Read the model definition and answer for the solid it produces. Units are mm, in the model's axes. Coordinates: 2 decimals unless noted, no trailing zeros. Order: outer loops, then holes, each group sorted by start corner. A loop starts at its lowest first (then second) coordinate and runs counter-clockwise, first axis right, second up.
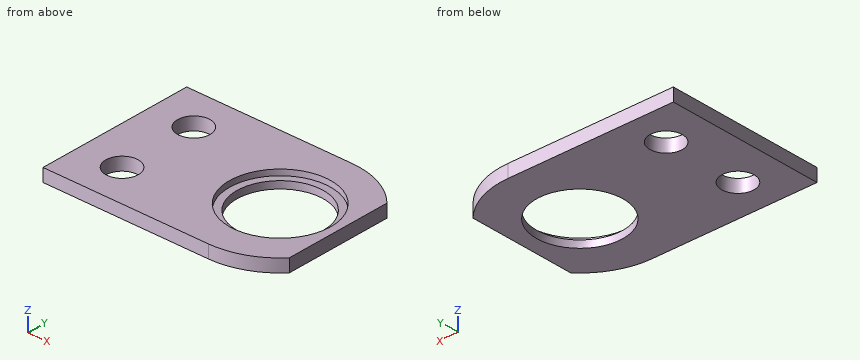
```python
from build123d import *

# Parameters (mm, degrees)
SKETCH_1_R          = 2.25
SKETCH_1_R_2        = 6
EXTRUDE_1_DEPTH     = 1.8
SKETCH_2_R          = 7
CUT_EXTRUDE_1_DEPTH = 0.8


with BuildPart() as part:
    # 草图1 → 凸台-拉伸1 (new body)
    with BuildSketch(Plane.XY):
        with BuildLine():
            Line((0, 7.478796414), (0, -7.478796414))
            ThreePointArc((0, -7.478796414), (-3.665697116, -10.081338219), (-8.066449293, -11))
            Line((-8.066449293, -11), (-31.066449293, -11))
            Line((-31.066449293, -11), (-31.066449293, 11))
            Line((-31.066449293, 11), (-8.066449293, 11))
            ThreePointArc((-8.066449293, 11), (-3.665697116, 10.081338219), (0, 7.478796414))
        make_face()
        with Locations((-25.066449293, 5.5)):
            Circle(SKETCH_1_R, mode=Mode.SUBTRACT)
        with Locations((-25.066449293, -5.5)):
            Circle(SKETCH_1_R, mode=Mode.SUBTRACT)
        with Locations((-8.066449293, 0)):
            Circle(SKETCH_1_R_2, mode=Mode.SUBTRACT)
    extrude(amount=EXTRUDE_1_DEPTH)

    # 草图2 → 切除-拉伸1 (cut)
    with BuildSketch(Plane.XY.offset(1.8)):
        with Locations((-8.066449293, 0)):
            Circle(SKETCH_2_R)
    extrude(amount=-CUT_EXTRUDE_1_DEPTH, mode=Mode.SUBTRACT)


solid = part.part
```
1) A cutting plane is placed at D-D, the plane y = 5. Determine the outline of the cut face in (x, z).
A:
outline: (-31.07, 0) - (-27.26, 0) - (-27.26, 1.8) - (-31.07, 1.8) - close; (-22.87, 0) - (-11.38, 0) - (-11.38, 1) - (-12.97, 1) - (-12.97, 1.8) - (-22.87, 1.8) - close; (-4.75, 0) - (0, 0) - (0, 1.8) - (-3.17, 1.8) - (-3.17, 1) - (-4.75, 1) - close
2) Straight lines are drawn through the part: line 1 (Y direction, x = -25.5, z = 1.35); line 2 (X direction, y = 5.75, z = 1.1); line 3 (X direction, y = 3.75, z = 0.25). For each, find the intervals that lie inside material, in ascending order.
A:
line 1: y = -11 to -7.71, -3.29 to 3.29, 7.71 to 11
line 2: x = -31.07 to -27.3, -22.83 to -12.06, -4.07 to 0
line 3: x = -31.07 to -26.48, -23.65 to -12.75, -3.38 to 0
3) A cutting plane is placed at B-B, the plane z = 0.5. Determine the outline of the cut face in (x, y).
A:
outline: (-31.07, -11) - (-8.07, -11) arc R11 ccw to (0, -7.48) - (0, 7.48) arc R11 ccw to (-8.07, 11) - (-31.07, 11) - close; hole circle Ø4.5 at (-25.07, -5.5); hole circle Ø4.5 at (-25.07, 5.5); hole circle Ø12 at (-8.07, 0)
4) A flat-ended cylindrical pin translates along its axis: pin 1 Ø7 at (x, y) = (-8.07, 0) entering from -Z. Find the tip coordinate at first contact, or state that the pin passes through.
A:
pin 1: passes through
5) A cutting plane is placed at A-A, the plane y = 0. Determine the outline of the cut face in (x, z).
A:
outline: (-31.07, 0) - (-14.07, 0) - (-14.07, 1) - (-15.07, 1) - (-15.07, 1.8) - (-31.07, 1.8) - close; (-2.07, 0) - (0, 0) - (0, 1.8) - (-1.07, 1.8) - (-1.07, 1) - (-2.07, 1) - close
6) A cutting plane is placed at C-C, the plane x = -9.5. Determine the outline of the cut face in (y, z).
A:
outline: (-11, 0) - (-5.83, 0) - (-5.83, 1) - (-6.85, 1) - (-6.85, 1.8) - (-11, 1.8) - close; (5.83, 0) - (11, 0) - (11, 1.8) - (6.85, 1.8) - (6.85, 1) - (5.83, 1) - close
